Here's the drawing with two shaded views (mm, measured from the low corner). I have some questions. A direction names the side the tool comes from. Give positions to 0.01 mm unless a question says otherwise; leave off trailing zeros. Order: outer loops, then holes, each group sorted by start corner. A loop starts at its lowest first (then second) coordinate and runs counter-clockwise, first axis right, second up. Notation, with made-up numbers: M 21,9.25 L 42,9.25 A25 cw 42,30.25 Z; hole C 37,48.5 d5. An arc over 180 degrees is marked long. Use a Markdown table: item, result. Add a question column.
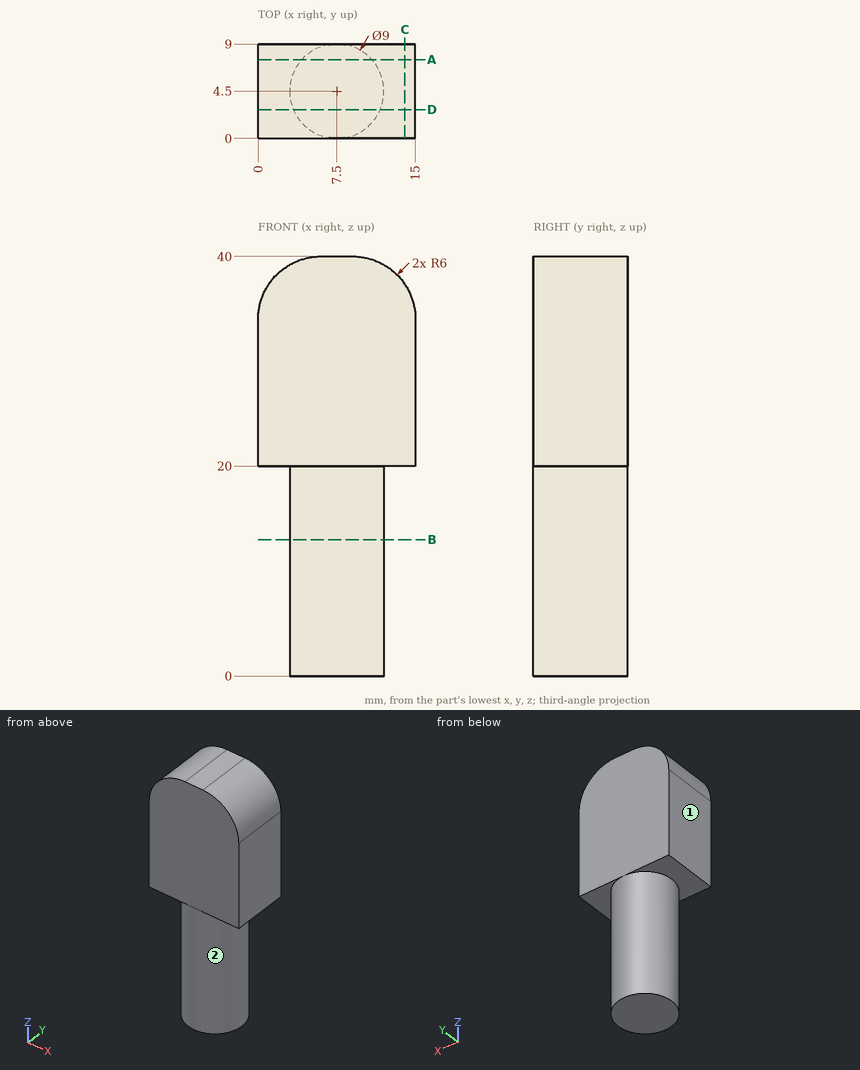
1) Suppose I cut it at A-A on y = 7.5. Please give me the cut outline in (x, z), and give its area (3 significant figures).
2) Suppose I cut it at C-C on x = 14. Please give me the cut outline in (y, z).
3) Suppose I cut it at B-B on z = 13. Please give me the cut outline in (x, y), and give its area (3 significant figures).
4) For pin 1 (4 mm diameter, centred on x = 8.5, z = 12.5, fed in from +Y); pin 2 (1.5 mm diameter, centred on x = 10, y = 6.5, fed in from +Z); pin 3 (4 mm diameter, centred on x = 13.5, y = 4, fed in from +Z); pin 4 (2 mm diameter, centred on y = 2, z = 8, fed in from +X), each with a flat end and sliding along its axis, tell me the tip position at first contact or that it passes through.
5) For the marked faces 1 and 2, which set-ups out of +Z, -Z, +X, -X, +Y, -Y let a thin tool reach every point of the face, with its end or its side?
6) Please list where these lines run through material, in increasing order: line 1 (Y direction, x = 10.25, z = 13.5); line 2 (X direction, y = 4.5, z = 16.5); line 3 (X direction, y = 8, z = 36). Write a range as from..to.
7) Suppose I cut it at D-D on y = 2.75. Please give me the cut outline in (x, z), and give its area (3 significant figures).
Values found:
| question | item | result |
|---|---|---|
| 1 | outline | M 0,20 L 4.15,20 L 4.15,0 L 10.85,0 L 10.85,20 L 15,20 L 15,34 A6 ccw 9,40 L 6,40 A6 ccw 0,34 Z |
| 1 | area | 419 mm^2 |
| 2 | outline | M 0,20 L 9,20 L 9,37.32 L 0,37.32 Z |
| 3 | outline | C 7.5,4.5 d9 |
| 3 | area | 63.6 mm^2 |
| 4 | pin 1 | stops at y = 9 |
| 4 | pin 2 | stops at z = 39.99 |
| 4 | pin 3 | stops at z = 39.45 |
| 4 | pin 4 | stops at x = 11.74 |
| 5 | face 1 | +Z, -Z, -X, +Y, -Y |
| 5 | face 2 | -Z |
| 6 | line 1 | y = 0.94..8.06 |
| 6 | line 2 | x = 3..12 |
| 6 | line 3 | x = 0.34..14.66 |
| 7 | outline | M 0,20 L 3.35,20 L 3.35,0 L 11.65,0 L 11.65,20 L 15,20 L 15,34 A6 ccw 9,40 L 6,40 A6 ccw 0,34 Z |
| 7 | area | 450 mm^2 |
